```python
from build123d import *

# Parameters (mm, degrees)
SKETCH1_W           = 23.5
SKETCH1_H           = 12.5
BOSS_EXTRUDE1_DEPTH = 2


with BuildPart() as part:
    # Sketch1 → Boss-Extrude1 (new body)
    with BuildSketch(Plane.YZ):
        Polygon((15.84119162, -7.151864849), (15.84119162, -8.348913545), (-15.15732803, -8.348913545), (-15.15732803, -6.848913545), (-15.15732803, 5.651086455), (-15.15732803, 7.151086455), (15.84119162, 7.151086455), (15.84119162, 6.848135151), align=None)
        with Locations((0.341931795, -0.598913545)):
            Rectangle(SKETCH1_W, SKETCH1_H, mode=Mode.SUBTRACT)
    extrude(amount=BOSS_EXTRUDE1_DEPTH)


solid = part.part
```
Check sheet for the modelled part. Datum: model origin and axes. Units: mm. A direction names the side the tool comes from. Give positions to 0.01 mm unless a question says otherwise; leave off trailing zeros. Order: outer loops, then holes, each group sorted by start corner. A loop starts at its lowest first (then second) coordinate and runs counter-clockwise, first axis right, second up. Notation, with made-up numbers: (8.25, 6) -> (23.25, 6) arc R27 ccw to (23.25, 32) -> close; hole circle Ø2 at (65, 4). An arc over 180 degrees is marked (long way). Use CSV: the item, a comma, the result in double quotes. Start each with the question number.
1) Sectioned sample at A-A, the plane z = 2. Record the boundary of the cut face in (x, y).
2) Go/stop test with flat-tipped pins: P1, Ø4, axis at y = -10, z = -3, coming from the +X side; P2, Ø1.5, axis at y = 6, z = -4.5, coming from the +X side. Record where each tip stops, or that it passes through.
3) Sectioned sample at B-B, the plane y = 1. Record the boundary of the cut face in (x, z), plus the area to 3 significant figures.
4) Set-up check for faces 1 (the face through (1, 12.092, -1)), 2 (the face through (2, 1, -7)): record each of +Z, -Z, +X, -X, +Y, -Y from which the full face is reachable in a straight line by a thin tool's end or side.
5) Material ranges on line 1 (Z direction, x = 1.9, y = -8); line 2 (Y direction, x = 0.1, z = 1.25), recorded low to high. Write a range as from..to.
6) Mould release check, pull along Y, two halves, no side actions. Record for faces 3 (the face through (1, 0, 7.151)), 4 (the face through (1, 0, 5.651)), 5 (the face through (1, 15.841, -1)): released by +Y, released by -Y, zero draft, split by the parting line, or undercut.
7) Sectioned sample at C-C, the plane x = 0.35. Record the boundary of the cut face in (y, z).
Recorded:
1,outline,"(0, -15.16) -> (2, -15.16) -> (2, -11.41) -> (0, -11.41) -> close; (0, 12.09) -> (2, 12.09) -> (2, 15.84) -> (0, 15.84) -> close"
2,P1,"x = 2"
2,P2,"through"
3,outline,"(0, -8.35) -> (2, -8.35) -> (2, -6.85) -> (0, -6.85) -> close; (0, 5.65) -> (2, 5.65) -> (2, 7.15) -> (0, 7.15) -> close"
3,area,"6.00 mm2"
4,face 1,"+X, -X"
4,face 2,"+Z, -Z, +X, +Y, -Y"
5,line 1,"-8.35..-6.85, 5.65..7.15"
5,line 2,"-15.16..-11.41, 12.09..15.84"
6,face 3,"zero draft"
6,face 4,"undercut"
6,face 5,"released by +Y"
7,outline,"(-15.16, -8.35) -> (15.84, -8.35) -> (15.84, 7.15) -> (-15.16, 7.15) -> close; hole (-11.41, -6.85) -> (12.09, -6.85) -> (12.09, 5.65) -> (-11.41, 5.65) -> close"
